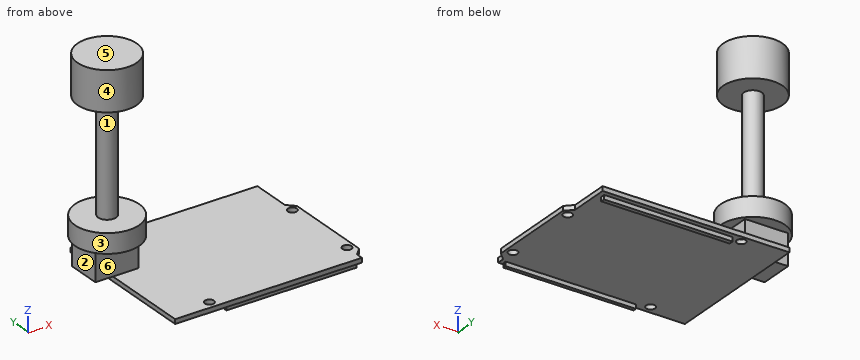
```python
from build123d import *

# Parameters (mm, degrees)
F0_R      = 1.6
F1_DEPTH  = 1.6
F2_W      = 6.2
F2_H      = 12
F2_W_2    = 9.04
F3_DEPTH  = 10.9
F4_W      = 46.085651
F4_H      = 1.150087
F4_W_2    = 45.428462
F4_H_2    = 1.478683
F5_DEPTH  = 1.5
F6_R      = 11.350572
F6_R_2    = 3.232045
F7_DEPTH  = 6.858
F8_R      = 3.175
F9_DEPTH  = 39.37
F10_R     = 10.465691
F10_R_2   = 3.175
F11_DEPTH = 13.97


with BuildPart() as f1:
    # F0 (on Top) → F1 (new body)
    with BuildSketch(Plane.XY):
        Polygon((0, 53.34), (0, 0), (66.04, 0), (66.04, 2.54), (68.58, 5.08), (68.58, 36.83), (66.04, 39.37), (66.04, 53.34), align=None)
        with Locations((14.14, 2.92)):
            Circle(F0_R, mode=Mode.SUBTRACT)
        with Locations((66.04, 7.62)):
            Circle(F0_R, mode=Mode.SUBTRACT)
        with Locations((15.24, 50.8)):
            Circle(F0_R, mode=Mode.SUBTRACT)
        with Locations((66.04, 35.56)):
            Circle(F0_R, mode=Mode.SUBTRACT)
    extrude(amount=F1_DEPTH)

    # F2 (on face) → F3 (join)
    with BuildSketch(Plane.XY.offset(1.6)):
        with Locations((-3.1, 37.74)):
            Rectangle(F2_W, F2_H)
        with Locations((4.52, 37.74)):
            Rectangle(F2_W_2, F2_H)
    extrude(amount=F3_DEPTH)

    # F4 (on face) → F5 (join)
    with BuildSketch(Plane(origin=(0, 0, 0), x_dir=(1, 0, 0), z_dir=(0, 0, -1))):
        with Locations((41.58383, -1.216432)):
            Rectangle(F4_W, F4_H)
        with Locations((41.611146, -50.914244)):
            Rectangle(F4_W_2, F4_H_2)
    extrude(amount=F5_DEPTH)

    # F6 (on face) → F7 (join)
    with BuildSketch(Plane.XY.offset(12.5)):
        with Locations((1.441258, 36.791712)):
            Circle(F6_R)
        with Locations((1.441258, 36.791712)):
            Circle(F6_R_2, mode=Mode.SUBTRACT)
        with Locations((1.441258, 36.791712)):
            Circle(F6_R_2)
    extrude(amount=F7_DEPTH)

    # F8 (on face) → F9 (join)
    with BuildSketch(Plane.XY.offset(19.358)):
        with Locations((1.441258, 36.791712)):
            Circle(F8_R)
    extrude(amount=F9_DEPTH)

    # F10 (on face) → F11 (join)
    with BuildSketch(Plane.XY.offset(58.728)):
        with Locations((1.441258, 36.791712)):
            Circle(F10_R)
        with Locations((1.441258, 36.791712)):
            Circle(F10_R_2)
    extrude(amount=F11_DEPTH)


solid = f1.part
```
Model file for the job. Use its own axes, mm. Face numbers are marked on the shaded views. A direction names the side the tool comes from. Coordinates: 2 decimals unless noted, no trailing zeros. Loops run counter-clockwise (first coordinate to the right, second up) from the corner with the lowest first, then second, coordinate; pieces in that order, holes last. Notation, with made-up numbers: (79, 81) - (83, 81) arc R14 cw to (83, 92) - close; hole circle Ø1 at (66.5, 17.25). An arc over 180 degrees is marked (long way). Write item = value, one per line. Start each with the question number.
Item 1: Wall check: probe 1 along Y at (x, z) = (15.24, 0.4); probe 2 along Z at (x, y) = (33.5, 42.5); probe 3 along Y at (x, z) = (8, 10.5). Give the ranges that are in metal, low to high. Write a range as [from, to].
Item 2: Pull direction Z, two halves, no side cores. Call the marked faces 4, 5 and 6: +Z half, -Z half, draft (parallel to the pull), parting line (faces both ways), or undercut.
Item 3: Saw through at B-B, the plane x = 20. List the corners of the cut face in (y, z), then the cut area to 3 significant figures.
Item 4: Saw through at A-A, the plane y = 7.62. List the corners of the cut face in (x, z), then the cut area to 3 significant figures.
Item 5: Drop flat-ended pins along their axis: pin 1 Ø18 at (x, y) = (1.5, 36) entering from -Z; pin 2 Ø0.8 at (x, z) = (43, -1) entering from -Y; pin 3 Ø8.5 at (y, z) = (36, 8) entering from +X; pin 4 Ø3 at (x, y) = (15.24, 50.8) entering from +Z. Give the stop position or say it passes through.
Item 6: Saw through at C-C, the plane y = 29. List the corners of the cut face in (x, z).
Item 7: Saw through at D-D, the plane z = 3. List the corners of the cut face in (x, y).
Item 8: 3-axis set-ups, long thin cutter, end or side, ignore diameter. For the marked faces 1, 2 and 3: which of +Z, -Z, +X, -X, +Y, -Y reach the whole face in a straight line?
Answers:
q1.probe_1 = [0, 1.76], [4.08, 49.2], [52.4, 53.34]
q1.probe_2 = [0, 1.6]
q1.probe_3 = [31.74, 43.74]
q2.face_4 = draft
q2.face_5 = +Z half
q2.face_6 = undercut
q3.outline = (0, 0) - (0.64, 0) - (0.64, -1.5) - (1.79, -1.5) - (1.79, 0) - (50.17, 0) - (50.17, -1.5) - (51.65, -1.5) - (51.65, 0) - (53.34, 0) - (53.34, 1.6) - (0, 1.6) - close
q3.area = 89.3 mm2
q4.outline = (0, 0) - (64.44, 0) - (64.44, 1.6) - (0, 1.6) - close; (67.64, 0) - (68.58, 0) - (68.58, 1.6) - (67.64, 1.6) - close
q4.area = 105 mm2
q5.pin_1 = 0
q5.pin_2 = 0.64
q5.pin_3 = 9.04
q5.pin_4 = through
q6.outline = (-6.81, 12.5) - (9.7, 12.5) - (9.7, 19.36) - (-6.81, 19.36) - close; (-5.55, 58.73) - (8.43, 58.73) - (8.43, 72.7) - (-5.55, 72.7) - close; (0, 0) - (68.58, 0) - (68.58, 1.6) - (0, 1.6) - close
q7.outline = (-6.2, 31.74) - (9.04, 31.74) - (9.04, 43.74) - (-6.2, 43.74) - close
q8.face_1 = none
q8.face_2 = -Z, -X, +Y, -Y
q8.face_3 = +Z
